CAD build for the part. Positions are in the model's coordinates, mm. A direction names the side the tool comes from. Give positions to 0.01 mm unless a question says otherwise; leave off trailing zeros. Write each loop counter-clockwise with the first axis right and the second up, starting at its lowest first coordinate (ties: lowest second). Pieces come first, ordered by that corner, then holes. Notation, with made-up numbers: (46, 47) - (91, 47) arc R6 ccw to (91, 54) - close; hole circle Ø9 at (66.25, 40.5). An arc over 180 degrees is marked (long way). Answer as a JSON object with one key per item and string values.
from build123d import *

# Parameters (mm, degrees)
SKETCH_1_R          = 1.5
SKETCH_1_R_2        = 1.75
EXTRUDE_1_DEPTH     = 3
FILLET_1_R          = 5
SKETCH_3_R          = 0.5
CUT_EXTRUDE_1_DEPTH = 10
SKETCH_4_R          = 4.05
CUT_EXTRUDE_2_DEPTH = 10
FILLET_2_R          = 1


with BuildPart() as part:
    # 草图1 → 凸台-拉伸1 (new body)
    with BuildSketch(Plane.XY):
        with BuildLine():
            Line((48.25, -17.561563803), (48.25, 0))
            ThreePointArc((48.25, 0), (45.781945765, 15.234038926), (38.630271835, 28.909593528))
            Line((38.630271835, 28.909593528), (28.062669438, 10.605969263))
            ThreePointArc((28.062669438, 10.605969263), (7.764571353, -28.977774789), (-29.605969263, -4.846295906))
            Line((-29.605969263, -4.846295906), (-46.660254038, 5))
            Line((-46.660254038, 5), (-60, 5))
            Line((-60, 5), (-60, -20.45))
            Line((-60, -20.45), (-48, -20.45))
            Line((-48, -20.45), (-48, -28.65))
            Line((-48, -28.65), (-52.5, -28.65))
            Line((-52.5, -28.65), (-52.5, -56.25))
            Line((-52.5, -56.25), (-29.605969263, -56.25))
            Line((-29.605969263, -56.25), (15.786547457, -56.25))
            Line((15.786547457, -56.25), (48.25, -17.561563803))
        make_face()
        with Locations((-45, -51.25)):
            Circle(SKETCH_1_R, mode=Mode.SUBTRACT)
        with Locations((-10, -51.25)):
            Circle(SKETCH_1_R, mode=Mode.SUBTRACT)
        with Locations((-55, -15.45)):
            Circle(SKETCH_1_R, mode=Mode.SUBTRACT)
        with Locations((-31.466251763, -31.466251763)):
            Circle(SKETCH_1_R_2, mode=Mode.SUBTRACT)
        with Locations((10, -51.25)):
            Circle(SKETCH_1_R, mode=Mode.SUBTRACT)
        with Locations((0, -42.5)):
            Circle(SKETCH_1_R_2, mode=Mode.SUBTRACT)
        with Locations((31.466251763, -31.466251763)):
            Circle(SKETCH_1_R_2, mode=Mode.SUBTRACT)
        with Locations((-55, -0.45)):
            Circle(SKETCH_1_R, mode=Mode.SUBTRACT)
        with Locations((-44.5, 0)):
            Circle(SKETCH_1_R_2, mode=Mode.SUBTRACT)
        with Locations((44.5, 0)):
            Circle(SKETCH_1_R_2, mode=Mode.SUBTRACT)
    extrude(amount=EXTRUDE_1_DEPTH)

    # 圆角1
    fillet_1_edges = [part.edges().sort_by_distance(p)[0] for p in [
        (48.25, -17.561563803, 1.5),
        (-46.660254038, 5, 1.5),
        (-29.605969263, -4.846295906, 1.5),
        (28.062669438, 10.605969263, 1.5),
        (38.630271835, 28.909593528, 1.5),
    ]]
    fillet(fillet_1_edges, radius=FILLET_1_R)

    # 草图3 → 切除-拉伸1 (cut)
    with BuildSketch(Plane(origin=(0, 0, 0), x_dir=(-1, 0, 0), z_dir=(0, 0, -1))):
        with Locations((48, -20.45)):
            Circle(SKETCH_3_R)
        with Locations((48, -28.65)):
            Circle(SKETCH_3_R)
    extrude(amount=-CUT_EXTRUDE_1_DEPTH, mode=Mode.SUBTRACT)

    # 草图4 → 切除-拉伸2 (cut)
    with BuildSketch(Plane.XY.offset(3)):
        with Locations((-20, -48.75)):
            Circle(SKETCH_4_R)
    extrude(amount=-CUT_EXTRUDE_2_DEPTH, mode=Mode.SUBTRACT)

    # 圆角2
    fillet_2_edges = [part.edges().sort_by_distance(p)[0] for p in [
        (15.786547457, -56.25, 1.5),
        (-52.5, -56.25, 1.5),
        (-52.5, -28.65, 1.5),
        (-60, -20.45, 1.5),
        (-60, 5, 1.5),
    ]]
    fillet(fillet_2_edges, radius=FILLET_2_R)


solid = part.part
Item 1: Cut at B-B (y = -8). Give the cut face in (x, z), and give its area (3 significant figures).
Entries:
{"outline": "(-60, 0) - (-28.91, 0) - (-28.91, 3) - (-60, 3) - close; (28.91, 0) - (48.25, 0) - (48.25, 3) - (28.91, 3) - close", "area": "151 mm2"}
Item 2: Cut at C-C (x = 44.5). Give the cut face in (y, z), and give its area (3 significant figures).
Entries:
{"outline": "(-22.03, 0) - (-1.75, 0) - (-1.75, 3) - (-22.03, 3) - close; (1.75, 0) - (18.65, 0) - (18.65, 3) - (1.75, 3) - close", "area": "112 mm2"}
Item 3: Cut at D-D (y = -51.25). Give the cut face in (x, z).
Entries:
{"outline": "(-52.5, 0) - (-46.5, 0) - (-46.5, 3) - (-52.5, 3) - close; (-43.5, 0) - (-23.19, 0) - (-23.19, 3) - (-43.5, 3) - close; (-16.81, 0) - (-11.5, 0) - (-11.5, 3) - (-16.81, 3) - close; (-8.5, 0) - (8.5, 0) - (8.5, 3) - (-8.5, 3) - close; (11.5, 0) - (19.98, 0) - (19.98, 3) - (11.5, 3) - close"}
Item 4: Mould opens along X. For faces 1 (the cylindrical face through (-53.57, 0, 1.48)), 2 (the flat face through (-52.5, -42, 1)), 3 (the flat face through (-53, 5, 1)) say: +X half, -X half, draft (parallel to the pull), parting line (faces both ways), or undercut.
Entries:
{"face 1": "undercut", "face 2": "-X half", "face 3": "draft"}
Item 5: Which spindle directions (+Z, -Z, +X, -X, +Y, -Y) get a long thin tool onto all of the face, cutting with end or side? Do faces 4 (the cylindrical face through (-42.883, -0.67, 1.479)), 5 (the flat face through (-38, 0, 1)), 6 (the flat face through (-50, -28.65, 1)). Say none if no direction does.
Entries:
{"face 4": "+Z, -Z", "face 5": "+Z, -Z, +Y", "face 6": "+Z, -Z, -X"}
Item 6: Probe line 1 (X direction, y = -15, z = 1.7); line 2 (X direction, y = -9, z = 0.3); line 3 (X direction, y = -22.5, z = 1.55). List the from-to ranges inside material, lowest first. Write a range as from..to.
Entries:
{"line 1": "-60..-56.43, -53.57..-25.98, 25.98..48.25", "line 2": "-60..-28.62, 28.62..48.25", "line 3": "-48..-19.84, 19.84..44.11"}
Item 7: Cut at A-A (x = -55). Give the cut face in (y, z), and give its area (4 significant figures).
Entries:
{"outline": "(-20.45, 0) - (-16.95, 0) - (-16.95, 3) - (-20.45, 3) - close; (-13.95, 0) - (-1.95, 0) - (-1.95, 3) - (-13.95, 3) - close; (1.05, 0) - (5, 0) - (5, 3) - (1.05, 3) - close", "area": "58.35 mm2"}
Item 8: Flat gauge pins, fed straight in: P1, Ø1.5, axis at x = -32, z = 0.5, coming from the +Y side; P2, Ø1.5, axis at y = 10, z = 2.5, coming from the -X side. Where does each tip first touch, or does it go through?
Entries:
{"P1": "y = -3.03", "P2": "x = 28.52"}
